```python
from build123d import *

# Parameters (mm, degrees)
CROQUIS1_W              = 40
CROQUIS1_H              = 40
SALIENTE_EXTRUIR1_DEPTH = 20
CROQUIS2_W              = 20
CROQUIS2_H              = 20
SALIENTE_EXTRUIR2_DEPTH = 20
SALIENTE_EXTRUIR3_DEPTH = 20


with BuildPart() as part:
    # Croquis1 → Saliente-Extruir1 (new body)
    with BuildSketch(Plane(origin=(0, 0, 0), x_dir=(1, 0, 0), z_dir=(0, 1, 0))):
        Rectangle(CROQUIS1_W, CROQUIS1_H)
    extrude(amount=SALIENTE_EXTRUIR1_DEPTH)

    # Croquis2 → Saliente-Extruir2 (add)
    with BuildSketch(Plane(origin=(0, 20, 0), x_dir=(1, 0, 0), z_dir=(0, 1, 0))):
        with Locations((-10, 10)):
            Rectangle(CROQUIS2_W, CROQUIS2_H)
    extrude(amount=SALIENTE_EXTRUIR2_DEPTH)

    # Croquis3 → Saliente-Extruir3 (add)
    with BuildSketch(Plane(origin=(20, 0, 0), x_dir=(0, 0, -1), z_dir=(1, 0, 0))):
        Polygon((20, 20), (20, 40), (0, 20), align=None)
    extrude(amount=-SALIENTE_EXTRUIR3_DEPTH)


solid = part.part
```
Work out the finished part from the listing and answer in its coordinate system (mm). A direction names the side the tool comes from. Give positions to 0.01 mm unless a question says otherwise; leave off trailing zeros. Loops run counter-clockwise (first coordinate to the right, second up) from the corner with the lowest first, then second, coordinate; pieces in that order, holes last. Notation, with made-up numbers: (-24, 45.5) -> (-2, 45.5) arc R20 ccw to (-2, 49.5) -> close; hole circle Ø4 at (-21.75, 74.5). An arc over 180 degrees is marked (long way). Write item = value, one per line. Start each with the question number.
(1) Find section A-A on z = -7. Give the vertices of the cut face in (x, y), and give its area (3 significant figures).
(2) Which of the six approach directions +Z, -Z, +X, -X, +Y, -Y give full straight-line access (tool end or side, diameter ignored) to faces 1 (the flat face through (0, 0, 0)), 2 (the flat face through (0, 34, -5)), 3 (the flat face through (-10, 30, 0))?
(3) Find section C-C on x = 17. Give the vertices of the cut face in (y, z), and give its area (3 significant figures).
(4) Find section B-B on y = 34.5. Give the vertices of the cut face in (x, z), and give its area (3 significant figures).
(5) Find section D-D on z = 12.5. Give the vertices of the cut face in (x, y).
(6) Given pin 1 Ø6 at (x, y) = (-12.5, 27.5) entering from +Z; pin 2 Ø6 at (x, z) = (-6.5, 5.5) entering from +Y; pin 3 Ø12 at (x, z) = (1, 3.5) entering from -Y; pin 4 Ø5 at (x, z) = (4.5, -5.5) entering from +Y, each flat-ended and moving along its own axis, determine where each tip first touches the part or whether it passes through.
(7) Find the intervals of material crossed by probe 1 along Y at (x, z) = (18, 9); probe 2 along Z at (x, y) = (-9.5, 29); probe 3 along Y at (x, z) = (13, -13.5), in increasing order. Write a range as from..to.
From the geometry:
q1.outline = (-20, 0) -> (20, 0) -> (20, 27) -> (0, 27) -> (0, 40) -> (-20, 40) -> close
q1.area = 1,340 mm^2
q2.face_1 = +Z, -Z, +X, -X, -Y
q2.face_2 = +Z, +X, +Y
q2.face_3 = +Z, +X, -X, +Y
q3.outline = (0, -20) -> (40, -20) -> (20, 0) -> (20, 20) -> (0, 20) -> close
q3.area = 1,000 mm^2
q4.outline = (-20, -20) -> (20, -20) -> (20, -14.5) -> (0, -14.5) -> (0, 0) -> (-20, 0) -> close
q4.area = 510 mm^2
q5.outline = (-20, 0) -> (20, 0) -> (20, 20) -> (-20, 20) -> close
q6.pin_1 = 0
q6.pin_2 = 20
q6.pin_3 = 0
q6.pin_4 = 28
q7.probe_1 = 0..20
q7.probe_2 = -20..0
q7.probe_3 = 0..33.5
